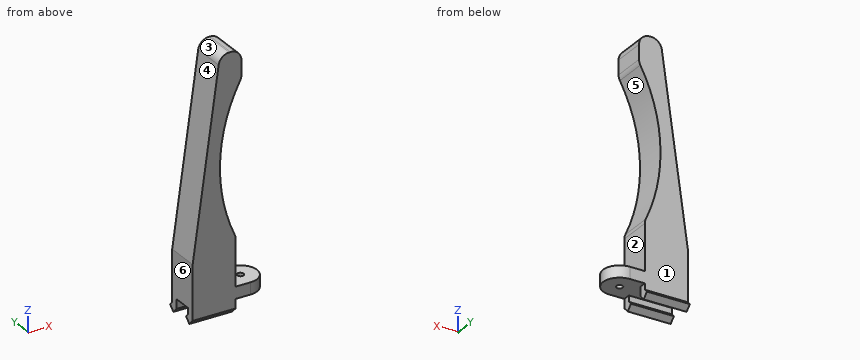
from build123d import *

# Parameters (mm, degrees)
SKETCH2_W           = 10
SKETCH2_H           = 14.768412439
BOSS_EXTRUDE1_DEPTH = 5
BOSS_EXTRUDE4_DEPTH = 10
SKETCH9_W           = 10
SKETCH9_H           = 3.18
SKETCH9_H_2         = 3.888412439
CUT_EXTRUDE3_DEPTH  = 5
BOSS_EXTRUDE5_DEPTH = 7.7
SKETCH12_R          = 0.75
BOSS_EXTRUDE7_DEPTH = 2.75
FILLET1_R           = 2.5


with BuildPart() as part:
    # Sketch2 → Boss-Extrude1 (new body)
    with BuildSketch(Plane.XY):
        with Locations((0, 1.566049366)):
            Rectangle(SKETCH2_W, SKETCH2_H)
    extrude(amount=BOSS_EXTRUDE1_DEPTH)

    # Sketch8 → Boss-Extrude4 (add)
    with BuildSketch(Plane.ZY.offset(5)):
        Polygon((-0.15, 5.770255585), (0, 5.770255585), (0, 4.070255585), (-0.15, 4.070255585), (-2.137867966, 4.070255585), (-3.402081528, 5.334469147), (-2.2, 6.536550675), (-1.43370491, 5.770255585), align=None)
        Polygon((-0.15, -1.929744415), (0, -1.929744415), (0, -0.229744415), (-0.15, -0.229744415), (-1.43370491, -0.229744415), (-2.2, 0.536550675), (-3.402081528, -0.665530853), (-2.137867966, -1.929744415), align=None)
    extrude(amount=-BOSS_EXTRUDE4_DEPTH)

    # Sketch9 → Cut-Extrude3 (cut)
    with BuildSketch(Plane(origin=(0, 0, 0), x_dir=(-1, 0, 0), z_dir=(0, 0, -1))):
        with Locations((0, 7.360255585)):
            Rectangle(SKETCH9_W, SKETCH9_H)
        with Locations((0, -3.873950635)):
            Rectangle(SKETCH9_W, SKETCH9_H_2)
    extrude(amount=-CUT_EXTRUDE3_DEPTH, mode=Mode.SUBTRACT)

    # Sketch10 → Boss-Extrude5 (add)
    with BuildSketch(Plane(origin=(0, 5.770255585, 0), x_dir=(1, 0, 0), z_dir=(0, 1, 0))):
        with BuildLine():
            Line((-5, -5), (-5, -10.5))
            Line((-5, -10.5), (1.352445729, -55.7))
            Line((1.352445729, -55.7), (6.352445729, -55.7))
            Line((6.352445729, -55.7), (6.352445729, -49.2))
            ThreePointArc((6.352445729, -49.2), (1.383429579, -31.764936646), (5, -14))
            Line((5, -14), (5, -5))
            Line((5, -5), (-5, -5))
        make_face()
    extrude(amount=-BOSS_EXTRUDE5_DEPTH)

    # Sketch12 → Boss-Extrude7 (add)
    with BuildSketch(Plane.XY):
        with BuildLine():
            Line((5, 5.770255585), (8.5, 5.770255585))
            ThreePointArc((8.5, 5.770255585), (12.35, 1.920255585), (8.5, -1.929744415))
            Line((8.5, -1.929744415), (5, -1.929744415))
            Line((5, -1.929744415), (5, 5.770255585))
        make_face()
        with Locations((8.5, 1.920255585)):
            Circle(SKETCH12_R, mode=Mode.SUBTRACT)
    extrude(amount=BOSS_EXTRUDE7_DEPTH)

    # Fillet1
    fillet1_edges = [part.edges().sort_by_distance(p)[0] for p in [
        (6.352445729, 1.920255585, 49.2),
        (5, 1.920255585, 14),
        (1.352445729, 1.920255585, 55.7),
        (6.352445729, 1.920255585, 55.7),
    ]]
    fillet(fillet1_edges, radius=FILLET1_R)


solid = part.part
Build history of the part. All positions in model axes, mm. Face numbers are marked on the shaded views. A direction names the side the tool comes from. Coordinates: 2 decimals unless noted, no trailing zeros. Order: outer loops, then holes, each group sorted by start corner. A loop starts at its lowest first (then second) coordinate and runs counter-clockwise, first axis right, second up. Notation, with made-up numbers: (-25, 37) - (2, 37) arc R6 cw to (2, 47) - close; hole circle Ø4 at (-18, 6.25). An arc over 180 degrees is marked (long way). Put each result on its own line as item: value.
1. Saw through at C-C (z = 6). Write the cut outline in (x, y), and give its area (3 significant figures).
Answer sheet:
outline: (-5, -1.93) - (5, -1.93) - (5, 5.77) - (-5, 5.77) - close
area: 77.0 mm^2
2. Saw through at B-B (x = 0). Write the cut outline in (y, z).
Answer sheet:
outline: (-1.93, -2.14) - (-0.67, -3.4) - (0.54, -2.2) - (-0.23, -1.43) - (-0.23, 0) - (4.07, 0) - (4.07, -2.14) - (5.33, -3.4) - (6.54, -2.2) - (5.77, -1.43) - (5.77, 46.08) - (-1.93, 46.08) - close
3. Saw through at A-A (x = 5.5). Write the cut outline in (y, z).
Answer sheet:
outline: (-1.93, 0) - (5.77, 0) - (5.77, 2.75) - (-1.93, 2.75) - close; (-1.93, 47.61) - (5.77, 47.61) - (5.77, 55.08) - (-1.93, 55.08) - close
4. Saw through at D-D (z = 40.5). Write the cut outline in (x, y).
Answer sheet:
outline: (-0.78, -1.93) - (2.74, -1.93) - (2.74, 5.77) - (-0.78, 5.77) - close
5. Pull direction Z, two halves, no side cores. Call the marked faces 4, 5 and 6: pulls with the +Z half, pulls with the -Z half, needs draft (parallel to the pull), parting line crosses it, or undercut.
Answer sheet:
face 4: pulls with the +Z half
face 5: undercut
face 6: needs draft
6. Drop flat-ended pins along their axis: P1, Ø2, axis at x = 9.5, y = 0, coming from the +Z side; P2, Ø10, axis at x = 4.5, z = 48, coming from the +Y side; P3, Ø1, axis at y = 2, z = 51, coming from the +X side; P4, Ø1.5, axis at x = 6.5, z = 46.5, coming from the +Y side. Give the stop position or say it passes through.
Answer sheet:
P1: stops at z = 2.75
P2: stops at y = 5.77
P3: stops at x = 6.35
P4: passes through
7. Tool access for the marked faces 1, 2 and 3: list every direction of +Z, -Z, +X, -X, +Y, -Y with a clear straight run to the whole face (end or side of a thin tool).
Answer sheet:
face 1: +Z, +X, -X, +Y
face 2: +X, +Y, -Y
face 3: +Z, -X, +Y, -Y
8. Probe line 1 along Y through (x, z) = (8.5, 0.85); line 2 along Z through (x, y) = (7, -0.75); line 3 along Y through (x, z) = (-3.5, 7). List the from-to ranges inside material, lowest first. Write a range as [from, to].
Answer sheet:
line 1: y = [-1.93, 1.17], [2.67, 5.77]
line 2: z = [0, 2.75]
line 3: y = [-1.93, 5.77]
